from build123d import *

# Parameters (mm, degrees)
SKETCH1_W           = 160
SKETCH1_H           = 200
BOSS_EXTRUDE1_DEPTH = 3
SKETCH2_R           = 1.5
SKETCH2_W           = 25
SKETCH2_H           = 2.05
SKETCH2_W_2         = 2.05
SKETCH2_H_2         = 50
SKETCH2_H_3         = 30
SKETCH2_W_3         = 15
SKETCH2_H_4         = 15
SKETCH2_W_4         = 44
SKETCH2_W_5         = 4
SKETCH2_H_5         = 22
SKETCH2_W_6         = 3.05
SKETCH2_H_6         = 35
CUT_EXTRUDE1_DEPTH  = 3
SKETCH3_R           = 1.5
CUT_EXTRUDE2_DEPTH  = 129.097619025
SKETCH4_R           = 7.5
SKETCH4_R_2         = 1.5
SKETCH4_W           = 10
SKETCH4_H           = 80
SKETCH4_W_2         = 70
SKETCH4_H_2         = 10
CUT_EXTRUDE3_DEPTH  = 3
SKETCH5_R           = 1.5
CUT_EXTRUDE4_DEPTH  = 10
SKETCH6_R           = 1.5
SKETCH6_W           = 10
SKETCH6_H           = 11
CUT_EXTRUDE5_DEPTH  = 10


with BuildPart() as part:
    # Sketch1 → Boss-Extrude1 (new body)
    with BuildSketch(Plane(origin=(0, 0, 0), x_dir=(1, 0, 0), z_dir=(0, 1, 0))):
        Rectangle(SKETCH1_W, SKETCH1_H)
    extrude(amount=BOSS_EXTRUDE1_DEPTH)

    # Sketch2 → Cut-Extrude1 (cut)
    with BuildSketch(Plane(origin=(0, 3, 0), x_dir=(1, 0, 0), z_dir=(0, 1, 0))):
        with Locations(Location((-60, -90, 0), (0, 0, 270))):
            Circle(SKETCH2_R)
        with Locations(Location((60, -90, 0), (0, 0, 90))):
            Circle(SKETCH2_R)
        with Locations(Location((0, -10, 0), (0, 0, 270))):
            Circle(SKETCH2_R)
        with Locations(Location((-65, 85, 0), (0, 0, 270))):
            Circle(SKETCH2_R)
        with Locations(Location((65, 85, 0), (0, 0, 90))):
            Circle(SKETCH2_R)
        with Locations((27.5, -93.975)):
            Rectangle(SKETCH2_W, SKETCH2_H)
        with Locations((-27.5, -93.975)):
            Rectangle(SKETCH2_W, SKETCH2_H)
        with Locations((73.975, 0)):
            Rectangle(SKETCH2_W_2, SKETCH2_H_2)
        with Locations((-73.975, 0)):
            Rectangle(SKETCH2_W_2, SKETCH2_H_2)
        with Locations((71.975, 80)):
            Rectangle(SKETCH2_W_2, SKETCH2_H_3)
        with Locations((-30.5, 92.5)):
            Rectangle(SKETCH2_W_3, SKETCH2_H_4)
        with Locations((2, 93.975)):
            Rectangle(SKETCH2_W_4, SKETCH2_H)
        with Locations((-71.975, 80)):
            Rectangle(SKETCH2_W_2, SKETCH2_H_3)
        with Locations((-8, 60)):
            Rectangle(SKETCH2_W_5, SKETCH2_H_5)
        with Locations((13.525, 58.5)):
            Rectangle(SKETCH2_W_6, SKETCH2_H_6)
    extrude(amount=-CUT_EXTRUDE1_DEPTH, mode=Mode.SUBTRACT)

    # Sketch3 → Cut-Extrude2 (cut, through all)
    with BuildSketch(Plane(origin=(0, 3, 0), x_dir=(1, 0, 0), z_dir=(0, 1, 0))):
        with Locations(Location((-24.13, 9.6, 0), (0, 0, 270))):
            Circle(SKETCH3_R)
        with Locations(Location((24.13, 8.36, 0), (0, 0, 270))):
            Circle(SKETCH3_R)
        with Locations(Location((-24.13, -72.92, 0), (0, 0, 270))):
            Circle(SKETCH3_R)
        with Locations(Location((24.13, -66.57, 0), (0, 0, 270))):
            Circle(SKETCH3_R)
    extrude(amount=-CUT_EXTRUDE2_DEPTH, mode=Mode.SUBTRACT)

    # Sketch4 → Cut-Extrude3 (cut)
    with BuildSketch(Plane(origin=(0, 3, 0), x_dir=(1, 0, 0), z_dir=(0, 1, 0))):
        with Locations(Location((-48, 55, 0), (0, 0, 270))):
            Circle(SKETCH4_R)
        with Locations(Location((48, 55, 0), (0, 0, 90))):
            Circle(SKETCH4_R)
        with Locations(Location((-60, 89.5, 0), (0, 0, 270))):
            Circle(SKETCH4_R_2)
        with Locations(Location((60, 89.5, 0), (0, 0, 90))):
            Circle(SKETCH4_R_2)
        with Locations(Location((-65, 36, 0), (0, 0, 270))):
            Circle(SKETCH4_R_2)
        with Locations(Location((65, 36, 0), (0, 0, 90))):
            Circle(SKETCH4_R_2)
        with Locations((-45, -10)):
            Rectangle(SKETCH4_W, SKETCH4_H)
        with Locations((45, -10)):
            Rectangle(SKETCH4_W, SKETCH4_H)
        with Locations((0, -83)):
            Rectangle(SKETCH4_W_2, SKETCH4_H_2)
    extrude(amount=-CUT_EXTRUDE3_DEPTH, mode=Mode.SUBTRACT)

    # Sketch5 → Cut-Extrude4 (cut)
    with BuildSketch(Plane(origin=(0, 3, 0), x_dir=(1, 0, 0), z_dir=(0, 1, 0))):
        with Locations(Location((-74, -83, 0), (0, 0, 270))):
            Circle(SKETCH5_R)
        with Locations(Location((-74, -59, 0), (0, 0, 270))):
            Circle(SKETCH5_R)
        with Locations(Location((-45, -83, 0), (0, 0, 270))):
            Circle(SKETCH5_R)
        with Locations(Location((-45, -59, 0), (0, 0, 270))):
            Circle(SKETCH5_R)
        with Locations(Location((45, -83, 0), (0, 0, 270))):
            Circle(SKETCH5_R)
        with Locations(Location((45, -59, 0), (0, 0, 270))):
            Circle(SKETCH5_R)
        with Locations(Location((74, -83, 0), (0, 0, 270))):
            Circle(SKETCH5_R)
        with Locations(Location((74, -59, 0), (0, 0, 270))):
            Circle(SKETCH5_R)
        with Locations(Location((6, 90, 0), (0, 0, 270))):
            Circle(SKETCH5_R)
        with Locations(Location((6, 75, 0), (0, 0, 270))):
            Circle(SKETCH5_R)
        with Locations(Location((35.0050005, 90, 0), (0, 0, 270))):
            Circle(SKETCH5_R)
        with Locations(Location((35, 66.000000521, 0), (0, 0, 270))):
            Circle(SKETCH5_R)
    extrude(amount=-CUT_EXTRUDE4_DEPTH, mode=Mode.SUBTRACT)

    # Sketch6 → Cut-Extrude5 (cut)
    with BuildSketch(Plane(origin=(0, 3, 0), x_dir=(1, 0, 0), z_dir=(0, 1, 0))):
        with Locations(Location((-33.5, 68.3, 0), (0, 0, 270))):
            Circle(SKETCH6_R)
        with Locations(Location((7, 54, 0), (0, 0, 270))):
            Circle(SKETCH6_R)
        with Locations((-30, 60.5)):
            Rectangle(SKETCH6_W, SKETCH6_H)
    extrude(amount=-CUT_EXTRUDE5_DEPTH, mode=Mode.SUBTRACT)


solid = part.part
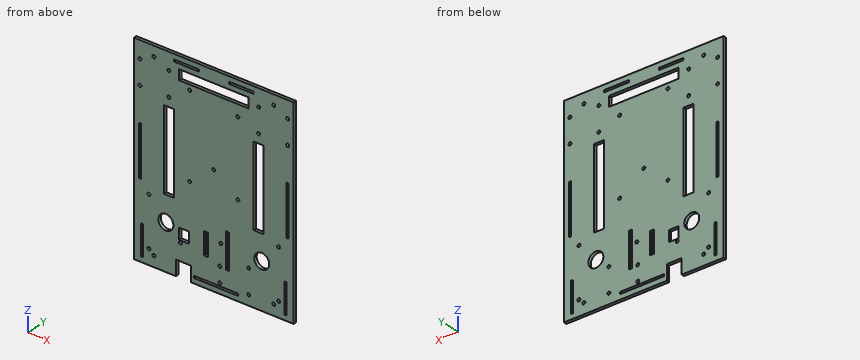
Part model, mm, in its own coordinate system. Round coordinates to 2 decimals unless told otherwise and drop trailing zeros. Loops run counter-clockwise (first coordinate to the right, second up) from the corner with the lowest first, then second, coordinate; pieces in that order, holes last. Notation, with made-up numbers: (26.5, 72.25) - (45.5, 72.25) arc R13 ccw to (45.5, 77.25) - close; hole circle Ø7 at (-6.75, -33.5). An arc over 180 degrees is marked (long way). Answer as a JSON object with one key per item and string values.
Item 1: Band-saw the part on A-A on z = 33.5. List the corners of the cut face in (x, y), plus the area to 3 significant figures.
Output:
{"outline": "(-80, 0) - (-50, 0) - (-50, 3) - (-80, 3) - close; (-40, 0) - (40, 0) - (40, 3) - (-40, 3) - close; (50, 0) - (80, 0) - (80, 3) - (50, 3) - close", "area": "420 mm2"}
Item 2: Band-saw the part on B-B on z = -59. List the corners of the cut face in (x, y), plus the area to 3 significant figures.
Output:
{"outline": "(-80, 0) - (-54.34, 0) - (-54.34, 3) - (-80, 3) - close; (-41.66, 0) - (-35, 0) - (-35, 3) - (-41.66, 3) - close; (-25, 0) - (-10, 0) - (-10, 3) - (-25, 3) - close; (-6, 0) - (12, 0) - (12, 3) - (-6, 3) - close; (15.05, 0) - (41.66, 0) - (41.66, 3) - (15.05, 3) - close; (54.34, 0) - (80, 0) - (80, 3) - (54.34, 3) - close", "area": "353 mm2"}
Item 3: Wall check: L1, parallel to X at y = 2, z = 83; L2, parallel to X at y = 1.2, z = -13.5; L3, parallel to Z at x = -13, y = 2.1. Give the ranges that are in metal, low to high.
Output:
{"L1": "-80 to -75.5, -72.5 to -46.5, -43.5 to -35, 35 to 43.5, 46.5 to 72.5, 75.5 to 80", "L2": "-80 to -75, -72.95 to -50, -40 to 40, 50 to 72.95, 75 to 80", "L3": "-100 to -95, -92.95 to 78, 88 to 100"}
Item 4: Band-saw the part on C-C on y = 1.6. State how many separate pieces and enclosed holes the cut face has, plus the area to 3 significant figures.
Output:
{"separate pieces": "1", "enclosed holes": "42", "area": "28,100 mm2"}
Item 5: Pin check, flat tips, straight feed: pin 1 (1.5 mm diameter, centred on x = 4, z = 18.5, fed in from -Y); pin 2 (1.5 mm diameter, centred on x = -27, y = 1.5, fed in from -Z). Stop position of each tip, or through.
Output:
{"pin 1": "y = 0", "pin 2": "z = -85"}
